```python
from build123d import *

# Parameters (mm, degrees)
SKETCH1_W       = 3
SKETCH1_H       = 2.5
EXTRUDE1_DEPTH  = 5
SKETCH2_W       = 0.645
SKETCH2_H       = 6
SKETCH2_H_2     = 3.5
EXTRUDE2_DEPTH  = 0.64
LPATTERN1_COUNT = 4
LPATTERN1_PITCH = 2.54
CHAMFER1_SIZE   = 0.25


with BuildPart() as part:
    # Sketch1 → Extrude1 (new, symmetric)
    with BuildSketch(Plane.XY):
        Rectangle(SKETCH1_W, SKETCH1_H)
    extrude(amount=EXTRUDE1_DEPTH, both=True)

    # Sketch2 → Extrude2 (add)
    with BuildSketch(Plane.XY.offset(3.86)):
        with Locations((0, 4.25)):
            Rectangle(SKETCH2_W, SKETCH2_H)
        with Locations((0, -3)):
            Rectangle(SKETCH2_W, SKETCH2_H_2)
    extrude2 = extrude(amount=-EXTRUDE2_DEPTH)

    # LPattern1: Extrude2 ×4
    with Locations(*[(0, 0, -i * LPATTERN1_PITCH) for i in range(1, LPATTERN1_COUNT)]):
        add(extrude2)

    # Chamfer1
    chamfer1_edges = [part.edges().sort_by_distance(p)[0] for p in [
        (0.3225, 7.25, 3.54),
        (0, 7.25, 3.22),
        (-0.3225, 7.25, 3.54),
        (0, 7.25, 3.86),
        (0, -4.75, 3.22),
        (0.3225, -4.75, 3.54),
        (-0.3225, -4.75, 3.54),
        (0, -4.75, 3.86),
        (0.3225, 7.25, 1),
        (0, 7.25, 0.68),
        (-0.3225, 7.25, 1),
        (0, 7.25, 1.32),
        (0, -4.75, 0.68),
        (0.3225, -4.75, 1),
        (-0.3225, -4.75, 1),
        (0, -4.75, 1.32),
        (0.3225, 7.25, -1.54),
        (0, 7.25, -1.86),
        (-0.3225, 7.25, -1.54),
        (0, 7.25, -1.22),
        (0, -4.75, -1.86),
        (0.3225, -4.75, -1.54),
        (-0.3225, -4.75, -1.54),
        (0, -4.75, -1.22),
        (0.3225, 7.25, -4.08),
        (0, 7.25, -4.4),
        (-0.3225, 7.25, -4.08),
        (0, 7.25, -3.76),
        (0, -4.75, -4.4),
        (0.3225, -4.75, -4.08),
        (-0.3225, -4.75, -4.08),
        (0, -4.75, -3.76),
    ]]
    chamfer(chamfer1_edges, length=CHAMFER1_SIZE)


solid = part.part
```
CAD build for the part. Positions are in the model's coordinates, mm. Coordinates: 2 decimals unless noted, no trailing zeros. Order: outer loops, then holes, each group sorted by start corner. A loop starts at its lowest first (then second) coordinate and runs counter-clockwise, first axis right, second up. Notation, with made-up numbers: (43.25, 15) - (87.25, 15) arc R14 cw to (87.25, 38) - close; hole circle Ø5 at (32, 10). An arc over 180 degrees is marked (long way). Use a Markdown table: item, result. Add a question column.
(1) Saw through at B-B (z = 1.5). Give the cut face in (x, y), then the cut area to 3 significant figures.
(2) Drill centre lines: line 1 along Y through (x, z) = (0.1, 3); line 2 along X through (y, z) = (2.5, 0.75). Where is each one in solid material? Low to high. Write a range as [from, to].
(3) Saw through at A-A (y = 2.5). Give the cut face in (x, z), then the cut area to 3 significant figures.
(4) Flat gauge pins, fed straight in: pin 1 (0.7 mm diameter, centred on x = 0, y = 3, fed in from +Z); pin 2 (0.5 mm diameter, centred on y = 3.5, z = 1, fed in from +X); pin 3 (1 mm diameter, centred on x = -1, z = -2, fed in from -Y). Where does each tip first touch, or does it go through?
(5) Saw through at C-C (x = 1.25). Give the cut face in (y, z), then the cut area to 3 significant figures.
Solved:
| question | item | result |
|---|---|---|
| 1 | outline | (-1.5, -1.25) - (1.5, -1.25) - (1.5, 1.25) - (-1.5, 1.25) - close |
| 1 | area | 7.50 mm² |
| 2 | line 1 | y = [-1.25, 1.25] |
| 2 | line 2 | x = [-0.32, 0.32] |
| 3 | outline | (-0.32, -4.4) - (0.32, -4.4) - (0.32, -3.76) - (-0.32, -3.76) - close; (-0.32, -1.86) - (0.32, -1.86) - (0.32, -1.22) - (-0.32, -1.22) - close; (-0.32, 0.68) - (0.32, 0.68) - (0.32, 1.32) - (-0.32, 1.32) - close; (-0.32, 3.22) - (0.32, 3.22) - (0.32, 3.86) - (-0.32, 3.86) - close |
| 3 | area | 1.65 mm² |
| 4 | pin 1 | stops at z = 3.86 |
| 4 | pin 2 | stops at x = 0.32 |
| 4 | pin 3 | stops at y = -1.25 |
| 5 | outline | (-1.25, -5) - (1.25, -5) - (1.25, 5) - (-1.25, 5) - close |
| 5 | area | 25.0 mm² |
